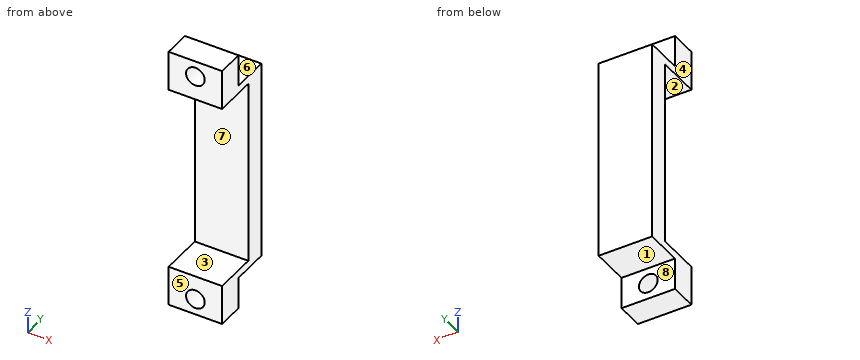
from build123d import *

# Parameters (mm, degrees)
CROQUIS1_W              = 40
CROQUIS1_H              = 50
SALIENTE_EXTRUIR1_DEPTH = 12
CROQUIS2_W              = 35
CROQUIS2_H              = 8
CORTAR_EXTRUIR1_DEPTH   = 65
CROQUIS3_W              = 30
CROQUIS3_H              = 50
CORTAR_EXTRUIR2_DEPTH   = 65
CROQUIS4_W              = 10
CROQUIS4_H              = 6
CORTAR_EXTRUIR3_DEPTH   = 7
CROQUIS5_R              = 1.75
CORTAR_EXTRUIR4_DEPTH   = 7


with BuildPart() as part:
    # Croquis1 → Saliente-Extruir1 (new body)
    with BuildSketch(Plane(origin=(0, 0, 0), x_dir=(1, 0, 0), z_dir=(0, 1, 0))):
        Rectangle(CROQUIS1_W, CROQUIS1_H)
    extrude(amount=SALIENTE_EXTRUIR1_DEPTH)

    # Croquis2 → Cortar-Extruir1 (cut)
    with BuildSketch(Plane(origin=(20, 0, 0), x_dir=(0, 0, -1), z_dir=(1, 0, 0))):
        with Locations((0, 4)):
            Rectangle(CROQUIS2_W, CROQUIS2_H)
    extrude(amount=-CORTAR_EXTRUIR1_DEPTH, mode=Mode.SUBTRACT)

    # Croquis3 → Cortar-Extruir2 (cut)
    with BuildSketch(Plane(origin=(0, 12, 0), x_dir=(1, 0, 0), z_dir=(0, 1, 0))):
        with Locations((-5, 0)):
            Rectangle(CROQUIS3_W, CROQUIS3_H)
    extrude(amount=-CORTAR_EXTRUIR2_DEPTH, mode=Mode.SUBTRACT)

    # Croquis4 → Cortar-Extruir3 (cut)
    with BuildSketch(Plane(origin=(0, 12, 0), x_dir=(1, 0, 0), z_dir=(0, 1, 0))):
        with Locations((15, 22)):
            Rectangle(CROQUIS4_W, CROQUIS4_H)
    cortar_extruir3 = extrude(amount=-CORTAR_EXTRUIR3_DEPTH, mode=Mode.SUBTRACT)

    # Simetría1: Cortar-Extruir3 across plane
    add(cortar_extruir3.mirror(Plane.XY), mode=Mode.SUBTRACT)

    # Croquis5 → Cortar-Extruir4 (cut)
    with BuildSketch(Plane(origin=(0, 5, 0), x_dir=(1, 0, 0), z_dir=(0, 1, 0))):
        with Locations(Location((15, 22, 0), (0, 0, 270))):
            Circle(CROQUIS5_R)
    cortar_extruir4 = extrude(amount=-CORTAR_EXTRUIR4_DEPTH, mode=Mode.SUBTRACT)

    # Simetría2: Cortar-Extruir4 across plane
    add(cortar_extruir4.mirror(Plane.XY), mode=Mode.SUBTRACT)


solid = part.part
The model under review builds one solid part; all positions refer to its coordinate system, in mm. Face numbers are marked on the shaded views. A direction names the side the tool comes from. Round coordinates to 2 decimals unless told otherwise and drop trailing zeros. Loops run counter-clockwise (first coordinate to the right, second up) from the corner with the lowest first, then second, coordinate; pieces in that order, holes last. Notation, with made-up numbers: (16, 83.5) - (59, 83.5) arc R18 cw to (59, 87.5) - close; hole circle Ø10 at (69.25, 55). An arc over 180 degrees is marked (long way). Use CSV: the item, a comma, the result in double quotes.
(1) Clearance check with flat-ended pins moving along their axes: P1, Ø3, axis at x = 13, z = 22.5, coming from the +Y side; P2, Ø2, axis at x = 14.5, y = 8.5, coming from the +Z side; P3, Ø3, axis at x = 12.5, z = -15, coming from the -Y side. State where each tip first meets the part, or that it passes through.
Working result:
P1,"stops at y = 5"
P2,"stops at z = 19"
P3,"stops at y = 8"
(2) Take a section at C-C, the plane x = 15. Give the boundary of the cut face in (y, z), plus the area to 3 significant figures.
Working result:
outline,"(0, -25) - (5, -25) - (5, -23.75) - (0, -23.75) - close; (0, -20.25) - (5, -20.25) - (5, -19) - (12, -19) - (12, 19) - (5, 19) - (5, 20.25) - (0, 20.25) - (0, 17.5) - (8, 17.5) - (8, -17.5) - (0, -17.5) - close; (0, 23.75) - (5, 23.75) - (5, 25) - (0, 25) - close"
area,"201 mm^2"
(3) For line 1 (Z direction, x = 14, y = 7); line 2 (X direction, y = 2.9, z = -22); line 3 (Z direction, x = 13.5, y = 1.75), list the stretches that pass through material, from the lowest coordinate up.
Working result:
line 1,"z = -19 to -17.5, 17.5 to 19"
line 2,"x = 10 to 13.25, 16.75 to 20"
line 3,"z = -25 to -22.9, -21.1 to -17.5, 17.5 to 21.1, 22.9 to 25"
(4) Take a section at B-B, the plane z = 22. Give the boundary of the cut face in (x, y), plus the area to 3 significant figures.
Working result:
outline,"(10, 0) - (13.25, 0) - (13.25, 5) - (10, 5) - close; (16.75, 0) - (20, 0) - (20, 5) - (16.75, 5) - close"
area,"32.5 mm^2"
(5) Take a section at A-A, the plane y = 2.5. Give the boundary of the cut face in (x, z), plus the area to 3 significant figures.
Working result:
outline,"(10, -25) - (20, -25) - (20, -17.5) - (10, -17.5) - close; (10, 17.5) - (20, 17.5) - (20, 25) - (10, 25) - close; hole circle Ø3.5 at (15, -22); hole circle Ø3.5 at (15, 22)"
area,"131 mm^2"
(6) Take a section at D-D, the plane y = 6. Give the boundary of the cut face in (x, z), plus the area to 3 significant figures.
Working result:
outline,"(10, -19) - (20, -19) - (20, -17.5) - (10, -17.5) - close; (10, 17.5) - (20, 17.5) - (20, 19) - (10, 19) - close"
area,"30.0 mm^2"
(7) The part is to be moulded in two halves that separate along Z. For the marked faces 1, 2, 3 and 4, say which applies: pulls with the +Z half, pulls with the -Z half, needs draft (parallel to the pull), parting line crosses it, or undercut.
Working result:
face 1,"pulls with the -Z half"
face 2,"undercut"
face 3,"undercut"
face 4,"needs draft"
(8) Machinability: for the marked faces 5, 6, 7 and 8, which of the approach directions +Z, -Z, +X, -X, +Y, -Y give a long, thin tool a straight path to every point of the face, cutting with its end or side? Answer none if there is none.
Working result:
face 5,"+Z, -Z, +X, -X, -Y"
face 6,"+Z, +X, -X, +Y"
face 7,"+X, -X, -Y"
face 8,"-Z, +X, -X, +Y"
